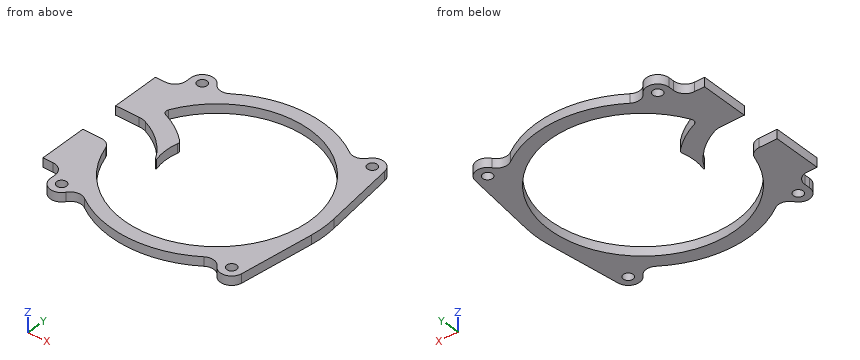
```python
from build123d import *

# Parameters (mm, degrees)
SKETCH_1_R      = 2.15
EXTRUDE_1_DEPTH = 4
FILLET_1_R      = 0.2
FILLET_2_R      = 2
FILLET_3_R      = 2
FILLET_4_R      = 8.5
FILLET_5_R      = 5


with BuildPart() as part:
    # 草图1 → 凸台-拉伸1 (new body)
    with BuildSketch(Plane.XY):
        with BuildLine():
            Line((-52, 8.75), (-52, 30))
            Line((-52, 30), (-47.54, 30))
            ThreePointArc((-47.54, 30), (-44.004466094, 31.464466094), (-42.54, 35))
            Line((-42.54, 35), (-42.54, 37.5))
            ThreePointArc((-42.54, 37.5), (-38.982425028, 42.287422066), (-33.372235985, 40.262198963))
            ThreePointArc((-33.372235985, 40.262198963), (-30.171244586, 38.118753147), (-26.396349665, 38.887436588))
            ThreePointArc((-26.396349665, 38.887436588), (0, 47), (26.396349665, 38.887436588))
            ThreePointArc((26.396349665, 38.887436588), (30.171244586, 38.118753147), (33.372235985, 40.262198963))
            ThreePointArc((33.372235985, 40.262198963), (38.674773042, 42.369526686), (42.499484755, 38.135225128))
            Line((42.499484755, 38.135225128), (46.619156699, 5.971116201))
            ThreePointArc((46.619156699, 5.971116201), (47, 0), (46.619156699, -5.971116201))
            Line((46.619156699, -5.971116201), (42.499484755, -38.135225128))
            ThreePointArc((42.499484755, -38.135225128), (38.674773042, -42.369526686), (33.372235985, -40.262198963))
            ThreePointArc((33.372235985, -40.262198963), (30.171244586, -38.118753147), (26.396349665, -38.887436588))
            ThreePointArc((26.396349665, -38.887436588), (0, -47), (-26.396349665, -38.887436588))
            ThreePointArc((-26.396349665, -38.887436588), (-30.171244586, -38.118753147), (-33.372235985, -40.262198963))
            ThreePointArc((-33.372235985, -40.262198963), (-38.982425028, -42.287422066), (-42.54, -37.5))
            Line((-42.54, -37.5), (-42.54, -35))
            ThreePointArc((-42.54, -35), (-44.004466094, -31.464466094), (-47.54, -30))
            Line((-47.54, -30), (-52, -30))
            Line((-52, -30), (-52, -8.75))
            Line((-52, -8.75), (-40.055430343, -8.75))
            ThreePointArc((-40.055430343, -8.75), (40.804364959, -4.000475011), (-37.593370285, 16.362717092))
            ThreePointArc((-37.593370285, 16.362717092), (-29.005163231, 12.290176631), (-21.585495377, 6.349518825))
            ThreePointArc((-21.585495377, 6.349518825), (-22.451945258, -1.469746278), (-20.573530425, -9.10932741))
            ThreePointArc((-20.573530425, -9.10932741), (-28.44850534, 1.855840669), (-40.055430343, 8.75))
            Line((-40.055430343, 8.75), (-52, 8.75))
        make_face()
        with Locations((-37.54, 37.5)):
            Circle(SKETCH_1_R, mode=Mode.SUBTRACT)
        with Locations((-37.54, -37.5)):
            Circle(SKETCH_1_R, mode=Mode.SUBTRACT)
        with Locations((37.54, -37.5)):
            Circle(SKETCH_1_R, mode=Mode.SUBTRACT)
        with Locations((37.54, 37.5)):
            Circle(SKETCH_1_R, mode=Mode.SUBTRACT)
    extrude(amount=EXTRUDE_1_DEPTH)

    # 圆角1
    fillet_1_edges = [part.edges().sort_by_distance(p)[0] for p in [
        (-20.573530425, -9.10932741, 2),
    ]]
    fillet(fillet_1_edges, radius=FILLET_1_R)

    # 圆角2
    fillet_2_edges = [part.edges().sort_by_distance(p)[0] for p in [
        (-21.585495377, 6.349518825, 2),
    ]]
    fillet(fillet_2_edges, radius=FILLET_2_R)

    # 圆角3
    fillet_3_edges = [part.edges().sort_by_distance(p)[0] for p in [
        (-37.593370285, 16.362717092, 2),
    ]]
    fillet(fillet_3_edges, radius=FILLET_3_R)

    # 圆角4
    fillet_4_edges = [part.edges().sort_by_distance(p)[0] for p in [
        (-40.055430343, 8.75, 2),
    ]]
    fillet(fillet_4_edges, radius=FILLET_4_R)

    # 圆角5
    fillet_5_edges = [part.edges().sort_by_distance(p)[0] for p in [
        (-40.055430343, -8.75, 2),
    ]]
    fillet(fillet_5_edges, radius=FILLET_5_R)


solid = part.part
```
Geometry check sheet. Reference: the model listing, model coordinates, mm. Round coordinates to 2 decimals unless told otherwise and drop trailing zeros. Loops run counter-clockwise (first coordinate to the right, second up) from the corner with the lowest first, then second, coordinate; pieces in that order, holes last. Notation, with made-up numbers: (74.25, 17) - (132.25, 17) arc R26 cw to (132.25, 41) - close; hole circle Ø5 at (-14.5, -30.5). An arc over 180 degrees is marked (long way). Use a Markdown table: item, result.
Q1. Cross-section at C-C on y = 33. Record the cut outline in (x, z), plus the area to 3 significant figures.
Solutions:
| item | result |
|---|---|
| outline | (-42.96, 0) - (-24.33, 0) - (-24.33, 4) - (-42.96, 4) - close; (24.33, 0) - (43.16, 0) - (43.16, 4) - (24.33, 4) - close |
| area | 150 mm2 |
Q2. Cross-section at A-A on x = -28.5. Record the cut outline in (y, z), plus the area to 3 significant figures.
Solutions:
| item | result |
|---|---|
| outline | (-38.07, 0) - (-29.47, 0) - (-29.47, 4) - (-38.07, 4) - close; (1.9, 0) - (11.97, 0) - (11.97, 4) - (1.9, 4) - close; (29.47, 0) - (38.07, 0) - (38.07, 4) - (29.47, 4) - close |
| area | 109 mm2 |
Q3. Go/stop test with flat-tipped pins: P1, Ø0.8, axis at y = 36.5, z = 1.5, coming from the -X side; P2, Ø2.5, axis at x = -37.54, y = -37.5, coming from the -Z side; P3, Ø1, axis at x = 16, z = 1, coming from the -Y side. Record where each tip stops, or that it passes through.
Solutions:
| item | result |
|---|---|
| P1 | stops at x = -42.54 |
| P2 | passes through |
| P3 | stops at y = -44.37 |
Q4. Cross-section at D-D on x = -16. Record the cut outline in (y, z), plus the area to 3 significant figures.
Solutions:
| item | result |
|---|---|
| outline | (-44.19, 0) - (-37.75, 0) - (-37.75, 4) - (-44.19, 4) - close; (37.75, 0) - (44.19, 0) - (44.19, 4) - (37.75, 4) - close |
| area | 51.5 mm2 |
Q5. Material ranges on line 1 (Y direction, x = 37.54, z = 2); line 2 (Y direction, x = -36.5, z = 3.65); line 3 (Y direction, x = -33, z = 3.3), recorded low to high.
Solutions:
| item | result |
|---|---|
| line 1 | y = -42.5 to -39.65, -35.35 to -16.48, 16.48 to 35.35, 39.65 to 42.5 |
| line 2 | y = -42.39 to -39.38, -35.62 to -18.67, 7.3 to 16.34, 18.67 to 35.62, 39.38 to 42.39 |
| line 3 | y = -39.77 to -24.33, 5.35 to 14.49, 24.33 to 39.77 |
Q6. Cross-section at B-B on x = 37.54. Record the cut outline in (y, z).
Solutions:
| item | result |
|---|---|
| outline | (-42.5, 0) - (-39.65, 0) - (-39.65, 4) - (-42.5, 4) - close; (-35.35, 0) - (-16.48, 0) - (-16.48, 4) - (-35.35, 4) - close; (16.48, 0) - (35.35, 0) - (35.35, 4) - (16.48, 4) - close; (39.65, 0) - (42.5, 0) - (42.5, 4) - (39.65, 4) - close |
